The model under review builds one solid part; all positions refer to its coordinate system, in mm. Face numbers are marked on the shaded views. A direction names the side the tool comes from. Give positions to 0.01 mm unless a question says otherwise; leave off trailing zeros. Loops run counter-clockwise (first coordinate to the right, second up) from the corner with the lowest first, then second, coordinate; pieces in that order, holes last. Notation, with made-up numbers: (-3.75, 70.25) - (54.25, 70.25) arc R18 ccw to (54.25, 97.25) - close; hole circle Ø11 at (-7.75, 17). An arc over 180 degrees is marked (long way). Return JSON: item names as keys, results as strings. Group by question number.
```python
from build123d import *

# Parameters (mm, degrees)
SKETCH1_W           = 23
SKETCH1_H           = 21.5
BOSS_EXTRUDE1_DEPTH = 12
SKETCH4_W           = 32
SKETCH4_H           = 12
BOSS_EXTRUDE2_DEPTH = 2
SKETCH5_R           = 5
BOSS_EXTRUDE3_DEPTH = 3
SKETCH6_R           = 2.5
BOSS_EXTRUDE4_DEPTH = 4
CUT_EXTRUDE1_DEPTH  = 4


with BuildPart() as part:
    # Sketch1 → Boss-Extrude1 (new body)
    with BuildSketch(Plane.XY):
        Rectangle(SKETCH1_W, SKETCH1_H)
    extrude(amount=BOSS_EXTRUDE1_DEPTH)

    # Sketch4 → Boss-Extrude2 (add)
    with BuildSketch(Plane(origin=(0, 6.75, 0), x_dir=(1, 0, 0), z_dir=(0, 1, 0))):
        with Locations((0, -6)):
            Rectangle(SKETCH4_W, SKETCH4_H)
    extrude(amount=-BOSS_EXTRUDE2_DEPTH)

    # Sketch5 → Boss-Extrude3 (add)
    with BuildSketch(Plane(origin=(0, 10.75, 0), x_dir=(1, 0, 0), z_dir=(0, 1, 0))):
        with Locations(Location((5.5, -6, 0), (0, 0, 270))):
            Circle(SKETCH5_R)
    extrude(amount=BOSS_EXTRUDE3_DEPTH)

    # Sketch6 → Boss-Extrude4 (add)
    with BuildSketch(Plane(origin=(0, 13.75, 0), x_dir=(1, 0, 0), z_dir=(0, 1, 0))):
        with Locations(Location((5.5, -6, 0), (0, 0, 270))):
            Circle(SKETCH6_R)
    extrude(amount=BOSS_EXTRUDE4_DEPTH)

    # Sketch7 → Cut-Extrude1 (cut)
    with BuildSketch(Plane(origin=(0, 6.75, 0), x_dir=(1, 0, 0), z_dir=(0, 1, 0))):
        with BuildLine():
            Line((-16, -4.178738648), (-14.337589365, -4.178738648))
            ThreePointArc((-14.337589365, -4.178738648), (-12.516328014, -6), (-14.337589365, -7.821261352))
            Line((-14.337589365, -7.821261352), (-16, -7.821261352))
            ThreePointArc((-16, -7.821261352), (-17.821261352, -6), (-16, -4.178738648))
        make_face()
        with BuildLine():
            Line((16, -4.178738648), (14.337589365, -4.178738648))
            ThreePointArc((14.337589365, -4.178738648), (12.516328014, -6), (14.337589365, -7.821261352))
            Line((14.337589365, -7.821261352), (16, -7.821261352))
            ThreePointArc((16, -7.821261352), (17.821261352, -6), (16, -4.178738648))
        make_face()
    extrude(amount=-CUT_EXTRUDE1_DEPTH, mode=Mode.SUBTRACT)


solid = part.part
```
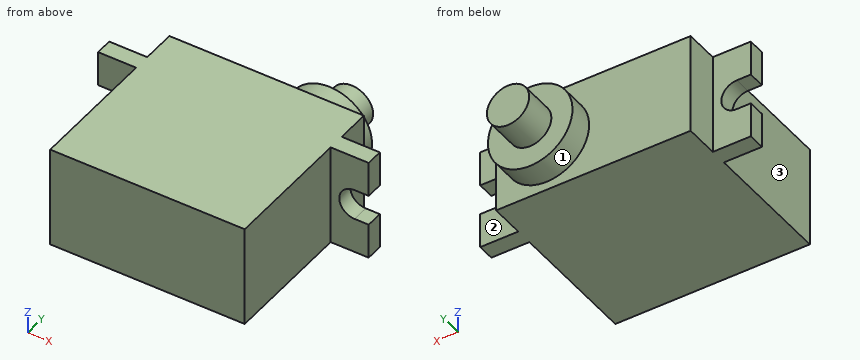
1) We need section C-C, the plane y = 3.5. Write out the cut boundary in (x, z).
2) For pin 1 Ø2 at (x, z) = (13.5, 8) entering from +Y; pin 2 Ø3.5 at (y, z) = (-1.5, 6.5) entering from -X; pin 3 Ø1 at (x, z) = (-1.5, 5.5) entering from +Y; pin 4 Ø4 at (x, y) = (-11.5, 0.5) entering from -Z, all flat-tipped, find the tip position at first contact; note any pin that passes through.
3) We need section B-B, the plane x = 5.5. Write out the cut boundary in (y, z).
4) Tool access review of the marked faces 1, 2 and 3: name each direction out of +Z, -Z, +X, -X, +Y, -Y from which nothing blocks a thin tool from reaching the whole face with its end or side.
5) To check wall thickness, follow line 1 (X direction, y = -5.5, z = 5.5); line 2 (Y direction, x = -6.5, z = 6); line 3 (Y direction, x = 13, z = 4). State the ranges of each line that lie inside material, in increasing order.
6) We need section A-A, the plane z = 6. Write out the cut boundary in (x, y).
7) We need section D-D, the plane z = 1.5. Write out the cut boundary in (x, y).
Findings:
{
 "1": {"outline": "(-11.5, 0) - (11.5, 0) - (11.5, 12) - (-11.5, 12) - close"},
 "2": {"pin 1": "stops at y = 6.75", "pin 2": "stops at x = -11.5", "pin 3": "stops at y = 10.75", "pin 4": "stops at z = 0"},
 "3": {"outline": "(-10.75, 0) - (10.75, 0) - (10.75, 1) - (13.75, 1) - (13.75, 3.5) - (17.75, 3.5) - (17.75, 8.5) - (13.75, 8.5) - (13.75, 11) - (10.75, 11) - (10.75, 12) - (-10.75, 12) - close"},
 "4": {"face 1": "+Y", "face 2": "+Z, -Z, +X, +Y", "face 3": "+Z, -Z, -X, -Y"},
 "5": {"line 1": "x = -11.5 to 11.5", "line 2": "y = -10.75 to 10.75", "line 3": "y = 4.75 to 6.75"},
 "6": {"outline": "(-12.52, 4.75) - (-11.5, 4.75) - (-11.5, -10.75) - (11.5, -10.75) - (11.5, 4.75) - (12.52, 4.75) - (12.52, 6.75) - (11.5, 6.75) - (11.5, 10.75) - (10.5, 10.75) - (10.5, 13.75) - (8, 13.75) - (8, 17.75) - (3, 17.75) - (3, 13.75) - (0.5, 13.75) - (0.5, 10.75) - (-11.5, 10.75) - (-11.5, 6.75) - (-12.52, 6.75) - close"},
 "7": {"outline": "(-16, 4.75) - (-11.5, 4.75) - (-11.5, -10.75) - (11.5, -10.75) - (11.5, 4.75) - (16, 4.75) - (16, 6.75) - (11.5, 6.75) - (11.5, 10.75) - (7.68, 10.75) - (7.68, 13.75) - (3.32, 13.75) - (3.32, 10.75) - (-11.5, 10.75) - (-11.5, 6.75) - (-16, 6.75) - close"}
}
